Build history of the part. All positions in model axes, mm. Round coordinates to 2 decimals unless told otherwise and drop trailing zeros. Write each loop counter-clockwise with the first axis right and the second up, starting at its lowest first coordinate (ties: lowest second). Pieces come first, ordered by that corner, then holes. Notation, with made-up numbers: (38.25, 27) -> (42.25, 27) arc R22 ccw to (42.25, 39) -> close; hole circle Ø1 at (51, 32.25). An arc over 180 degrees is marked (long way). Answer in a Markdown table with one row per item. Add a question column.
from build123d import *

# Parameters (mm, degrees)
SKETCH1_W           = 240
SKETCH1_H           = 130
SKETCH1_W_2         = 3.175
SKETCH1_H_2         = 4
SKETCH1_W_3         = 4
SKETCH1_H_3         = 3.175
SKETCH1_W_4         = 20
BOSS_EXTRUDE4_DEPTH = 3.175


with BuildPart() as part:
    # Sketch1 → Boss-Extrude4 (new body)
    with BuildSketch(Plane(origin=(0, 0, 0), x_dir=(1, 0, 0), z_dir=(0, 1, 0))):
        Rectangle(SKETCH1_W, SKETCH1_H)
        with Locations((-111.5875, 50)):
            Rectangle(SKETCH1_W_2, SKETCH1_H_2, mode=Mode.SUBTRACT)
        with Locations((-105, 56.5875)):
            Rectangle(SKETCH1_W_3, SKETCH1_H_3, mode=Mode.SUBTRACT)
        with Locations((105, 56.5875)):
            Rectangle(SKETCH1_W_3, SKETCH1_H_3, mode=Mode.SUBTRACT)
        with Locations((111.5875, 50)):
            Rectangle(SKETCH1_W_2, SKETCH1_H_2, mode=Mode.SUBTRACT)
        with Locations((-111.5875, -50)):
            Rectangle(SKETCH1_W_2, SKETCH1_H_2, mode=Mode.SUBTRACT)
        with Locations((-60, -56.5875)):
            Rectangle(SKETCH1_W_4, SKETCH1_H_3, mode=Mode.SUBTRACT)
        with Locations((111.5875, -50)):
            Rectangle(SKETCH1_W_2, SKETCH1_H_2, mode=Mode.SUBTRACT)
        with Locations((-100, -56.5875)):
            Rectangle(SKETCH1_W_4, SKETCH1_H_3, mode=Mode.SUBTRACT)
        with Locations((-20, -56.5875)):
            Rectangle(SKETCH1_W_4, SKETCH1_H_3, mode=Mode.SUBTRACT)
        with Locations((20, -56.5875)):
            Rectangle(SKETCH1_W_4, SKETCH1_H_3, mode=Mode.SUBTRACT)
        with Locations((60, -56.5875)):
            Rectangle(SKETCH1_W_4, SKETCH1_H_3, mode=Mode.SUBTRACT)
        with Locations((100, -56.5875)):
            Rectangle(SKETCH1_W_4, SKETCH1_H_3, mode=Mode.SUBTRACT)
        with Locations((-66.5, -23.4125)):
            Rectangle(SKETCH1_W_3, SKETCH1_H_3, mode=Mode.SUBTRACT)
        with Locations((-55, -23.4125)):
            Rectangle(SKETCH1_W_3, SKETCH1_H_3, mode=Mode.SUBTRACT)
        with Locations((-43.5, -23.4125)):
            Rectangle(SKETCH1_W_3, SKETCH1_H_3, mode=Mode.SUBTRACT)
        with Locations((43.5, -23.4125)):
            Rectangle(SKETCH1_W_3, SKETCH1_H_3, mode=Mode.SUBTRACT)
        with Locations((55, -23.4125)):
            Rectangle(SKETCH1_W_3, SKETCH1_H_3, mode=Mode.SUBTRACT)
        with Locations((66.5, -23.4125)):
            Rectangle(SKETCH1_W_3, SKETCH1_H_3, mode=Mode.SUBTRACT)
        with Locations((-11.5, -23.4125)):
            Rectangle(SKETCH1_W_3, SKETCH1_H_3, mode=Mode.SUBTRACT)
        with Locations((0, -23.4125)):
            Rectangle(SKETCH1_W_3, SKETCH1_H_3, mode=Mode.SUBTRACT)
        with Locations((11.5, -23.4125)):
            Rectangle(SKETCH1_W_3, SKETCH1_H_3, mode=Mode.SUBTRACT)
        with BuildLine():
            Line((-85, -36.438117734), (85, -36.438117734))
            ThreePointArc((85, -36.438117734), (90, -41.438117734), (85, -46.438117734))
            Line((85, -46.438117734), (-85, -46.438117734))
            ThreePointArc((-85, -46.438117734), (-90, -41.438117734), (-85, -36.438117734))
        make_face(mode=Mode.SUBTRACT)
    extrude(amount=BOSS_EXTRUDE4_DEPTH)


solid = part.part
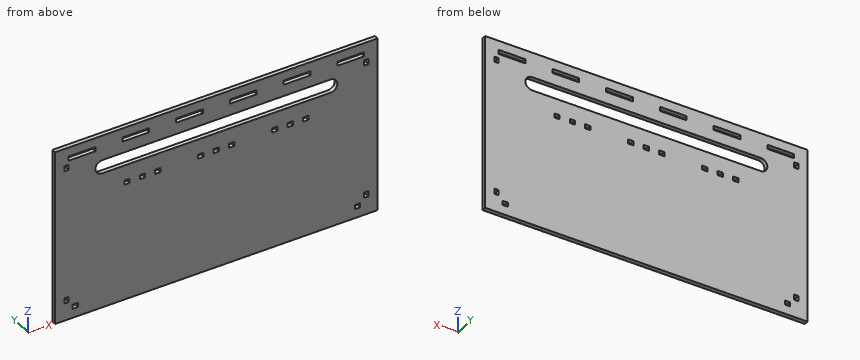
(1) Saw through at B-B (z = 42.5). List the corners of the cut face in (x, y) (3 decimals), plus the area to 3 significant figures.
(2) Probe line 1 along X through (y, z) = (0.9, -56.5); line 2 along Z through (x, y) = (-53.5, 2.9) (3 decimals); line 3 along Z through (x, y) = (-64, 2.2) (3 decimals). List the from-to ranges inside material, lowest first.
(3) Saw through at C-C (y = 1.25). Count the separate pieces of the cut face and the enclosed holes in it, plus the area to 4 significant figures.
(4) Saw through at A-A (x = -26). List the corners of the cut face in (y, z) (3 decimals).
Answer sheet:
| question | item | result |
|---|---|---|
| 1 | outline | (-120, 0) -> (-89.886, 0) -> (-89.886, 3.175) -> (-120, 3.175) -> close; (89.886, 0) -> (120, 0) -> (120, 3.175) -> (89.886, 3.175) -> close |
| 1 | area | 191 mm² |
| 2 | line 1 | x = -120 to -107, -103 to 103, 107 to 120 |
| 2 | line 2 | z = -65 to 21.825, 25 to 36.438, 46.438 to 55, 58.175 to 65 |
| 2 | line 3 | z = -65 to 36.438, 46.438 to 55, 58.175 to 65 |
| 3 | separate pieces | 1 |
| 3 | enclosed holes | 22 |
| 3 | area | 28,850 mm² |
| 4 | outline | (0, -65) -> (3.175, -65) -> (3.175, 36.438) -> (0, 36.438) -> close; (0, 46.438) -> (3.175, 46.438) -> (3.175, 55) -> (0, 55) -> close; (0, 58.175) -> (3.175, 58.175) -> (3.175, 65) -> (0, 65) -> close |
